from build123d import *

# Parameters (mm, degrees)
SKETCH1_R                           = 50.8
BOSS_EXTRUDE1_DEPTH                 = 82.55
F_1_4_20_TAPPED_HOLE1_D             = 5.1054
F_1_4_20_TAPPED_HOLE1_DEPTH         = 19.05
F_1_4_20_TAPPED_HOLE1_TIP           = 1.533816902
F_5_32_0_15625_DIAMETER_HOLE1_D     = 3.96875
F_5_32_0_15625_DIAMETER_HOLE1_DEPTH = 5.08
F_5_32_0_15625_DIAMETER_HOLE1_TIP   = 1.192332791


with BuildPart() as part:
    # Sketch1 → Boss-Extrude1 (new body)
    with BuildSketch(Plane(origin=(0, 0, 0), x_dir=(1, 0, 0), z_dir=(0, 1, 0))):
        Circle(SKETCH1_R)
    extrude(amount=BOSS_EXTRUDE1_DEPTH)

    # 1/4-20 Tapped Hole1
    with Locations(Plane(origin=(0, 0, 0), x_dir=(-1, 0, 0), z_dir=(0, -1, 0))):
        with Locations((0, 0)):
            Hole(F_1_4_20_TAPPED_HOLE1_D / 2, depth=F_1_4_20_TAPPED_HOLE1_DEPTH)
            with Locations((0, 0, -(F_1_4_20_TAPPED_HOLE1_DEPTH + F_1_4_20_TAPPED_HOLE1_TIP / 2))):  # 118° drill point
                Cone(0, F_1_4_20_TAPPED_HOLE1_D / 2, F_1_4_20_TAPPED_HOLE1_TIP, mode=Mode.SUBTRACT)

    # 5/32 (0.15625) Diameter Hole1
    with Locations(Plane(origin=(0, 0, 0), x_dir=(-1, 0, 0), z_dir=(0, -1, 0))):
        with Locations((0, 44.45), (0, -44.45)):
            Hole(F_5_32_0_15625_DIAMETER_HOLE1_D / 2, depth=F_5_32_0_15625_DIAMETER_HOLE1_DEPTH)
            with Locations((0, 0, -(F_5_32_0_15625_DIAMETER_HOLE1_DEPTH + F_5_32_0_15625_DIAMETER_HOLE1_TIP / 2))):  # 118° drill point
                Cone(0, F_5_32_0_15625_DIAMETER_HOLE1_D / 2, F_5_32_0_15625_DIAMETER_HOLE1_TIP, mode=Mode.SUBTRACT)


solid = part.part
Input: part model. Units: mm. Frame: model coordinates. A direction names the side the tool comes from. Round coordinates to 2 decimals unless told otherwise and drop trailing zeros. Loops run counter-clockwise (first coordinate to the right, second up) from the corner with the lowest first, then second, coordinate; pieces in that order, holes last. Notation, with made-up numbers: (26.25, 86.5) -> (66.25, 86.5) arc R7 ccw to (66.25, 95.5) -> close; hole circle Ø2 at (13.25, 36). An arc over 180 degrees is marked (long way). Answer as a JSON object with one key per item and string values. Group by question number.
1) Section query C-C on y = 47.5. Output: boundary loops of the cut face in (x, z), plus the area to 3 significant figures.
2) Draft query along Z for faces 1 (the conical face through (0, 6, -44)), 2 (the flat face through (11, 0, -1)), 3 (the cylindrical face through (-11.012, 40.697, 49.592)). Return one class per face: +Z half, -Z half, draft (parallel to the pull), parting line (faces both ways), or undercut.
3) Section query B-B on x = 30.5. Output: boundary loops of the cut face in (y, z) (3 decimals), plus the area to 3 significant figures.
4) Section query A-A on y = 17.5. Output: boundary loops of the cut face in (x, z), plus the area to 3 significant figures.
5) Section query D-D on x = -18. Output: boundary loops of the cut face in (y, z).
6) Reachability of faces 4 (the cylindrical face through (-0.43, 2.576, -42.513)), 5 (the flat face through (-1, 82.55, -1)) from +Z, -Z, +X, -X, +Y, -Y: full face, straight path, thin tool, end or side. Return the list, or none.
7) Pin query (flat end, axial travel): pin 1 (5 mm diameter, centred on x = -36.5, y = 43, fed in from +Z); pin 2 (4 mm diameter, centred on x = 16.5, y = 18.5, fed in from -Z); pin 3 (1.5 mm diameter, centred on y = 66, z = 25, fed in from +X). Return the tip coordinate at first contact, or that it passes through.
8) Ray query, L1, parallel to Z at x = 0, y = 1; L2, parallel to X at y = 2, z = 44.45; L3, parallel to X at y = 1, z = 44. Return the intervals inside material, ascending.
Reply:
{
 "1": {"outline": "circle Ø101.6 at (0, 0)", "area": "8,110 mm2"},
 "2": {"face 1": "undercut", "face 2": "draft", "face 3": "parting line"},
 "3": {"outline": "(0, -40.625) -> (82.55, -40.625) -> (82.55, 40.625) -> (0, 40.625) -> close", "area": "6,710 mm2"},
 "4": {"outline": "circle Ø101.6 at (0, 0); hole circle Ø5.11 at (0, 0)", "area": "8,090 mm2"},
 "5": {"outline": "(0, -47.5) -> (82.55, -47.5) -> (82.55, 47.5) -> (0, 47.5) -> close"},
 "6": {"face 4": "-Y", "face 5": "+Z, -Z, +X, -X, +Y"},
 "7": {"pin 1": "stops at z = 37.74", "pin 2": "stops at z = -48.69", "pin 3": "stops at x = 44.64"},
 "8": {"L1": "z = -50.8 to -46.43, -42.47 to -2.55, 2.55 to 42.47, 46.43 to 50.8", "L2": "x = -24.59 to -1.98, 1.98 to 24.59", "L3": "x = -25.39 to -1.93, 1.93 to 25.39"}
}
